For this review, take the finished solid that the model builds, in its own axes (mm). A direction names the side the tool comes from. Coordinates: 2 decimals unless noted, no trailing zeros. Loops run counter-clockwise (first coordinate to the right, second up) from the corner with the lowest first, then second, coordinate; pieces in that order, holes last.
Autodesk Inventor part; units mm, degrees
ref_plane "YZ Plane" through (0, 0, 0) normal (1, 0, 0) x (0, 1, 0)
ref_plane "XZ Plane" through (0, 0, 0) normal (0, 1, 0) x (-1, 0, 0)
ref_plane "XY Plane" through (0, 0, 0) normal (0, 0, 1) x (1, 0, 0)
sketch "Sketch1" plane through (0, 0, 0) normal (0, 1, 0) x (-1, 0, 0)
  circle A0 centre (0, 0) radius 5
  line L0 (-12, 13.25) -> (-12, -13.25)
  line L1 (-49.85, 0) -> (19.1, 0) construction
  arc A1 (-12, -21.25) -> (-12, 21.25) centre (-12, 0) ccw
  line L2 (-12, -21.25) -> (-40, -21.25)
  line L3 (-40, -21.25) -> (-40, -13.25)
  line L4 (-40, -13.25) -> (-12, -13.25)
  line L5 (-12, 21.25) -> (-40, 21.25)
  line L6 (-40, 21.25) -> (-40, 13.25)
  line L7 (-40, 13.25) -> (-12, 13.25)
  dimension "d0" = 10
  dimension "d1" = 42.5
  dimension "d2" = 12
  dimension "d3" = 8
  dimension "d4" = 28
  dimension "d5" = 21.25
extrude "Extrusion1" add sketch "Sketch1" along normal blind 15
properties part number "giunto_barra_estrusore"
Q1. Consider section D-D (x = 6). State the section outline as (y, z) points.
Q2. Consider section A-A (z = 0). State the section outline as (x, y) points, then the cut area to 3 significant figures.
Q3. For pin 1 Ø2 at (y, z) = (7.5, 2.5) entering from +X; pin 2 Ø5 at (y, z) = (3.5, 12) entering from -X, all flat-tipped, find the tip position at first contact; note any pin that passes through.
Q4. Consider section C-C (x = 34). State the section outline as (y, z) points, then the cut area to 3 significant figures.
Q5. Consider section B-B (y = 1). State the section outline as (x, z) points, then the cut area to 3 significant figures.
Q6. Machinability: for faces 1 (the face through (26, 7, 21.25)), 2 (the face through (26, 7, -13.25)), which of the approach directions +Z, -Z, +X, -X, +Y, -Y give a long, thin tool a straight path to every point of the face, cutting with its end or side? Answer none if there is none.
Q7. The part is to be moulded in two halves that separate along Z. For faces 3 (the face through (-9.245, 7.395, 0.467)), 4 (the face through (10, 0, 0)), 5 (the face through (1.08, 7.4, 4.88)), say which applies: +Z half, -Z half, draft (parallel to the pull), parting line (faces both ways), or undercut.
Q8. Wall thickness on probe 1 along Z at (x, y) = (21.5, 12.25); probe 2 along Z at (x, y) = (0, 9.25); probe 3 along X at (y, z) = (4.25, -15.5): over which ranges is each line inside the solid? List them lowest first.
Model answer:
1. outline: (0, -20.39) - (15, -20.39) - (15, 20.39) - (0, 20.39) - close
2. outline: (-9.25, 0) - (-5, 0) - (-5, 15) - (-9.25, 15) - close; (5, 0) - (12, 0) - (12, 15) - (5, 15) - close
2. area: 169 mm2
3. pin 1: stops at x = 12
3. pin 2: stops at x = -7.01
4. outline: (0, -21.25) - (15, -21.25) - (15, -13.25) - (0, -13.25) - close; (0, 13.25) - (15, 13.25) - (15, 21.25) - (0, 21.25) - close
4. area: 240 mm2
5. outline: (12, -21.25) - (40, -21.25) - (40, -13.25) - (12, -13.25) - (12, 13.25) - (40, 13.25) - (40, 21.25) - (12, 21.25) arc R21.25 ccw to start; hole circle Ø10 at (0, 0)
5. area: 1,080 mm2
6. face 1: +Z, +X, -X, +Y, -Y
6. face 2: +X, +Y, -Y
7. face 3: parting line
7. face 4: draft
7. face 5: undercut
8. probe 1: z = -21.25 to -13.25, 13.25 to 21.25
8. probe 2: z = -17.54 to -5, 5 to 17.54
8. probe 3: x = -2.54 to 40
